```python
from build123d import *

# Parameters (mm, degrees)
SKETCH_W            = 36.3
SKETCH_H            = 60
PAD_DEPTH           = 2.5
FILLET_R            = 8.23
FILLET001_R         = 11.5
HOLE_D              = 2.9
HOLE_DEPTH          = 25
HOLE_CSINK_D        = 6.1
HOLE_CSINK_ANGLE    = 90
SKETCH002_R         = 8.5
PAD001_DEPTH        = 2
SKETCH003_R         = 2.25
POCKET_DEPTH        = 2
HOLE001_D           = 3.4
HOLE001_DEPTH       = 25
HOLE001_CSINK_D     = 6.1
HOLE001_CSINK_ANGLE = 90


with BuildPart() as part:
    # Sketch → Pad (new body)
    with BuildSketch(Plane.XY):
        with Locations((0, 30)):
            Rectangle(SKETCH_W, SKETCH_H)
    extrude(amount=PAD_DEPTH)

    # Fillet
    fillet_edges = [part.edges().sort_by_distance(p)[0] for p in [
        (18.15, 0, 1.25),
        (-18.15, 0, 1.25),
    ]]
    fillet(fillet_edges, radius=FILLET_R)

    # Fillet001
    fillet001_edges = [part.edges().sort_by_distance(p)[0] for p in [
        (-18.15, 60, 1.25),
        (18.15, 60, 1.25),
    ]]
    fillet(fillet001_edges, radius=FILLET001_R)

    # Hole
    with Locations(Plane.XY.offset(2.5)):
        with Locations((0, 4), (-14.553, 14.594), (14.553, 14.594)):
            CounterSinkHole(HOLE_D / 2, HOLE_CSINK_D / 2, depth=HOLE_DEPTH, counter_sink_angle=HOLE_CSINK_ANGLE)

    # Sketch002 (on Face5 of Hole) → Pad001 (join)
    with BuildSketch(Plane.XY.offset(2.5)):
        with Locations((0, 48.5)):
            Circle(SKETCH002_R)
    extrude(amount=PAD001_DEPTH)

    # Sketch003 (on Face18 of Pad001) → Pocket (cut)
    with BuildSketch(Plane.XY.offset(4.5)):
        with Locations((0, 48.5)):
            Circle(SKETCH003_R)
    extrude(amount=-POCKET_DEPTH, mode=Mode.SUBTRACT)

    # Hole001
    with Locations(Plane(origin=(0, 0, 0), x_dir=(1, 0, 0), z_dir=(0, 0, -1))):
        with Locations((0, -48.5)):
            CounterSinkHole(HOLE001_D / 2, HOLE001_CSINK_D / 2, depth=HOLE001_DEPTH, counter_sink_angle=HOLE001_CSINK_ANGLE)


solid = part.part
```
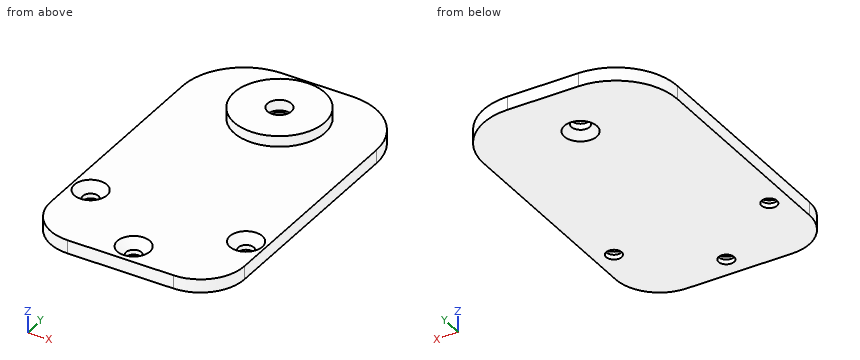
Work out the finished part from the listing and answer in its coordinate system (mm). Coordinates: 2 decimals unless noted, no trailing zeros. Write each loop counter-clockwise with the first axis right and the second up, starting at its lowest first coordinate (ties: lowest second). Pieces come first, ordered by that corner, then holes. Notation, with made-up numbers: (69, -11) - (102, -11) arc R20 cw to (102, 20) - close; hole circle Ø9 at (31.5, 79.25). An arc over 180 degrees is marked (long way). Answer as a JSON object with one key per item and string values.
Q1. Given pin 1 Ø1.5 at (x, y) = (14.5, 36.5) entering from -Z; pin 2 Ø1.7 at (x, y) = (14.553, 14.594) entering from +Z; pin 3 Ø8 at (x, y) = (-14.5, 26.5) entering from +Z, each flat-ended and moving along its own axis, determine where each tip first touches the part or whether it passes through.
Results list:
{"pin 1": "stops at z = 0", "pin 2": "passes through", "pin 3": "stops at z = 2.5"}
Q2. Find section D-D (y = 34.5). Write down the section's boundary in (x, z), plus the area to 4 significant figures.
Results list:
{"outline": "(-18.15, 0) - (18.15, 0) - (18.15, 2.5) - (-18.15, 2.5) - close", "area": "90.75 mm^2"}
Q3. Find section B-B (y = 4). Write down the section's boundary in (x, z).
Results list:
{"outline": "(-16.98, 0) - (-1.45, 0) - (-1.45, 0.9) - (-3.05, 2.5) - (-16.98, 2.5) - close; (1.45, 0) - (16.98, 0) - (16.98, 2.5) - (3.05, 2.5) - (1.45, 0.9) - close"}
Q4. Find section C-C (z = 3.1). Write down the section's boundary in (x, y), plus the area to 3 significant figures.
Results list:
{"outline": "circle Ø17 at (0, 48.5); hole circle Ø4.5 at (0, 48.5)", "area": "211 mm^2"}
Q5. Find section A-A (x = 0). Write down the section's boundary in (y, z).
Results list:
{"outline": "(0, 0) - (2.55, 0) - (2.55, 0.9) - (0.95, 2.5) - (0, 2.5) - close; (5.45, 0) - (45.45, 0) - (46.8, 1.35) - (46.8, 2.5) - (46.25, 2.5) - (46.25, 4.5) - (40, 4.5) - (40, 2.5) - (7.05, 2.5) - (5.45, 0.9) - close; (50.2, 1.35) - (51.55, 0) - (60, 0) - (60, 2.5) - (57, 2.5) - (57, 4.5) - (50.75, 4.5) - (50.75, 2.5) - (50.2, 2.5) - close"}
Q6. Consider L1, parallel to Y at x = 0, z = 3.95; L2, parallel to Z at x = 15.5, y = 35; L3, parallel to Y at x = 2, z = 0.5. Determine where each line is inside the solid, lowest interval first. Write a range as from..to.
Results list:
{"L1": "y = 40..46.25, 50.75..57", "L2": "z = 0..2.5", "L3": "y = 0..46.92, 50.08..60"}
